Verification items for the finished model (mm, model axes). Face numbers are marked on the shaded views. Coordinates: 2 decimals unless noted, no trailing zeros. Write each loop counter-clockwise with the first axis right and the second up, starting at its lowest first coordinate (ties: lowest second). Pieces come first, ordered by that corner, then holes. Notation, with made-up numbers: M -21,-20.5 L 26,-20.5 A24 cw 26,18.5 Z; hole C 18,89.25 d9. An arc over 180 degrees is marked long. Answer in a Markdown table with one row per item.
from build123d import *

# Parameters (mm, degrees)
SKETCH_1_W          = 75
SKETCH_1_H          = 40
EXTRUDE_1_DEPTH     = 4
SKETCH_3_R          = 3
CUT_EXTRUDE_1_DEPTH = 4
SKETCH_4_R          = 1.5
CUT_EXTRUDE_2_DEPTH = 10
FILLET_1_R          = 3
CUT_EXTRUDE_3_DEPTH = 10
EXTRUDE_2_DEPTH     = 4
FILLET_2_R          = 1.25


with BuildPart() as part:
    # 草图1 → 凸台-拉伸1 (new body)
    with BuildSketch(Plane.XY):
        Rectangle(SKETCH_1_W, SKETCH_1_H)
    extrude(amount=EXTRUDE_1_DEPTH)

    # 草图3 → 切除-拉伸1 (cut)
    with BuildSketch(Plane.XY.offset(4)):
        Circle(SKETCH_3_R)
    extrude(amount=-CUT_EXTRUDE_1_DEPTH, mode=Mode.SUBTRACT)

    # 草图4 → 切除-拉伸2 (cut)
    with BuildSketch(Plane.XY.offset(4)):
        with Locations((32.5, 15)):
            Circle(SKETCH_4_R)
        with Locations((-32.5, 15)):
            Circle(SKETCH_4_R)
        with Locations((-32.5, -15)):
            Circle(SKETCH_4_R)
        with Locations((32.5, -15)):
            Circle(SKETCH_4_R)
    extrude(amount=-CUT_EXTRUDE_2_DEPTH, mode=Mode.SUBTRACT)

    # 圆角1
    fillet_1_edges = [part.edges().sort_by_distance(p)[0] for p in [
        (37.5, -20, 2),
        (-37.5, -20, 2),
        (-37.5, 20, 2),
        (37.5, 20, 2),
    ]]
    fillet(fillet_1_edges, radius=FILLET_1_R)

    # 草图5 → 切除-拉伸3 (cut)
    with BuildSketch(Plane.XY.offset(4)):
        with BuildLine():
            Line((-29.5, 14), (-3, 14))
            Line((-3, 14), (-3, 6.873863542))
            ThreePointArc((-3, 6.873863542), (-7.5, 0), (-3, -6.873863542))
            Line((-3, -6.873863542), (-3, -14))
            Line((-3, -14), (-29.5, -14))
            Line((-29.5, -14), (-29.5, 14))
        make_face()
    cut_extrude_3 = extrude(amount=-CUT_EXTRUDE_3_DEPTH, mode=Mode.SUBTRACT)

    # 镜向1: 切除-拉伸3 across plane
    add(cut_extrude_3.mirror(Plane(origin=(0, 0, 0), x_dir=(0, 0, 1), z_dir=(1, 0, 0))), mode=Mode.SUBTRACT)

    # 草图6 → 凸台-拉伸2 (add)
    with BuildSketch(Plane.XY.offset(4)):
        with BuildLine():
            Line((-7.460046298, -0.773116571), (-29.5, -11.232755616))
            Line((-29.5, -11.232755616), (-29.5, -14))
            Line((-29.5, -14), (-23.669020762, -14))
            Line((-23.669020762, -14), (-5.316324036, -5.290245622))
            ThreePointArc((-5.316324036, -5.290245622), (-6.775693577, -3.215583392), (-7.460046298, -0.773116571))
        make_face()
        with BuildLine():
            Line((-29.5, 14), (-29.5, 11.232755616))
            Line((-29.5, 11.232755616), (-7.460046298, 0.773116571))
            ThreePointArc((-7.460046298, 0.773116571), (-6.775693577, 3.215583392), (-5.316324036, 5.290245622))
            Line((-5.316324036, 5.290245622), (-23.669020762, 14))
            Line((-23.669020762, 14), (-29.5, 14))
        make_face()
        with BuildLine():
            Line((23.669020762, 14), (5.316324036, 5.290245622))
            ThreePointArc((5.316324036, 5.290245622), (6.775693577, 3.215583392), (7.460046298, 0.773116571))
            Line((7.460046298, 0.773116571), (29.5, 11.232755616))
            Line((29.5, 11.232755616), (29.5, 14))
            Line((29.5, 14), (23.669020762, 14))
        make_face()
        with BuildLine():
            ThreePointArc((7.460046298, -0.773116571), (6.775693577, -3.215583392), (5.316324036, -5.290245622))
            Line((5.316324036, -5.290245622), (23.669020762, -14))
            Line((23.669020762, -14), (29.5, -14))
            Line((29.5, -14), (29.5, -11.232755616))
            Line((29.5, -11.232755616), (7.460046298, -0.773116571))
        make_face()
    extrude(amount=-EXTRUDE_2_DEPTH)

    # 圆角2
    fillet_2_edges = [part.edges().sort_by_distance(p)[0] for p in [
        (3, -14, 2),
        (3, -6.873863542, 2),
        (3, 6.873863542, 2),
        (3, 14, 2),
        (-29.5, -11.232755616, 2),
        (-7.460046298, -0.773116571, 2),
        (-5.316324036, -5.290245622, 2),
        (-23.669020762, -14, 2),
        (-23.669020762, 14, 2),
        (-5.316324036, 5.290245622, 2),
        (-7.460046298, 0.773116571, 2),
        (-29.5, 11.232755616, 2),
        (5.316324036, 5.290245622, 2),
        (23.669020762, 14, 2),
        (29.5, 11.232755616, 2),
        (7.460046298, 0.773116571, 2),
        (7.460046298, -0.773116571, 2),
        (29.5, -11.232755616, 2),
        (23.669020762, -14, 2),
        (5.316324036, -5.290245622, 2),
        (-3, 14, 2),
        (-3, 6.873863542, 2),
        (-3, -6.873863542, 2),
        (-3, -14, 2),
    ]]
    fillet(fillet_2_edges, radius=FILLET_2_R)


solid = part.part
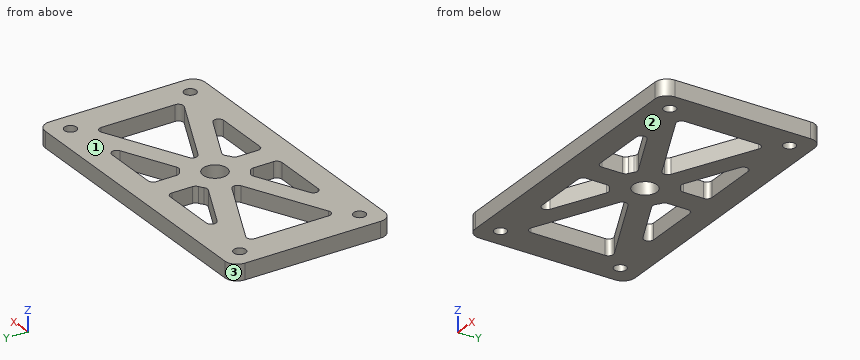
1) Thickness scan on L1, parallel to Y at x = -32.5, z = 2.6; L2, parallel to Y at x = 0, z = 2.75; L3, parallel to X at y = -11, z = 2.7. Record the ranges inside material, lowest first. Write a range as [from, to].
Response values:
| item | result |
|---|---|
| L1 | y = [-20, -16.5], [-13.5, 13.5], [16.5, 20] |
| L2 | y = [-20, -3], [3, 20] |
| L3 | x = [-37.5, -17.35], [-3, 3], [17.35, 37.5] |
2) Release check for a two-part mould opening along Z. For the marked faces 1, 2 and 3 record: +Z half, -Z half, draft (parallel to the pull), parting line (faces both ways), or undercut.
Response values:
| item | result |
|---|---|
| face 1 | +Z half |
| face 2 | -Z half |
| face 3 | draft |
3) Sectioned sample at B-B (x = 32.5). Record the cut outline in (y, z), then the cut area to 3 significant figures.
Response values:
| item | result |
|---|---|
| outline | M -20,0 L -16.5,0 L -16.5,4 L -20,4 Z; M -13.5,0 L 13.5,0 L 13.5,4 L -13.5,4 Z; M 16.5,0 L 20,0 L 20,4 L 16.5,4 Z |
| area | 136 mm² |
4) Sectioned sample at C-C (x = 0). Record the cut outline in (y, z), then the cut area to 3 significant figures.
Response values:
| item | result |
|---|---|
| outline | M -20,0 L -3,0 L -3,4 L -20,4 Z; M 3,0 L 20,0 L 20,4 L 3,4 Z |
| area | 136 mm² |
5) Sectioned sample at D-D (x = -17). Record the cut outline in (y, z), then the cut area to 3 significant figures.
Response values:
| item | result |
|---|---|
| outline | M -20,0 L -14,0 L -14,4 L -20,4 Z; M -10.84,0 L -5.3,0 L -5.3,4 L -10.84,4 Z; M 5.3,0 L 10.84,0 L 10.84,4 L 5.3,4 Z; M 14,0 L 20,0 L 20,4 L 14,4 Z |
| area | 92.3 mm² |
6) Depth check by flat-ended pin: pin 1 (3.5 mm diameter, centred on x = 0, y = 0, fed in from -Z); pin 2 (1.5 mm diameter, centred on x = -17.5, y = 11.5, fed in from -Z). Enter the tip coordinate at first touch or a pass-through.
Response values:
| item | result |
|---|---|
| pin 1 | passes through |
| pin 2 | stops at z = 0 |
7) Sectioned sample at A-A (y = 15). Record the cut outline in (x, z), then the cut area to 3 significant figures.
Response values:
| item | result |
|---|---|
| outline | M -37.5,0 L -34,0 L -34,4 L -37.5,4 Z; M -31,0 L 31,0 L 31,4 L -31,4 Z; M 34,0 L 37.5,0 L 37.5,4 L 34,4 Z |
| area | 276 mm² |
